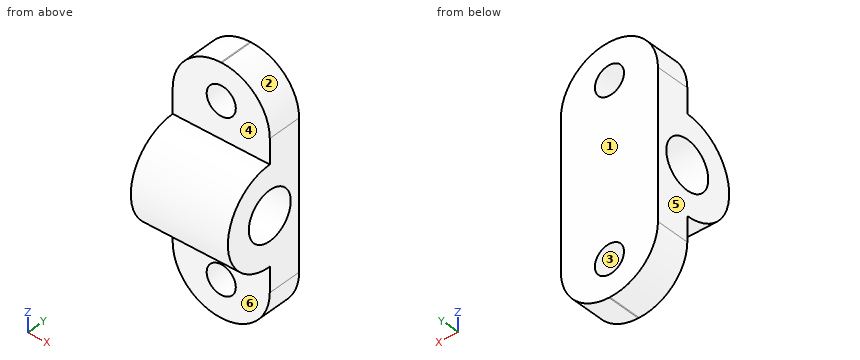
from build123d import *

# Parameters (mm, degrees)
PAD030_DEPTH             = 20
SKETCH021_R              = 5
POCKET001006_DEPTH       = 20.001
FILLET_R                 = 9.9
SKETCH024_R              = 3
POCKET002_DEPTH          = 7.001
CLONE076_ROLL_ANGLE      = 90
CLONE076_PLACEMENT_ANGLE = -90


with BuildPart() as part:
    # Sketch020 → Pad030 (new body)
    with BuildSketch(Plane.XY):
        with BuildLine():
            Line((18, 0), (25, 0))
            Line((25, 0), (25, 15))
            ThreePointArc((25, 15), (35, 25), (25, 35))
            Line((25, 35), (25, 50))
            Line((25, 50), (18, 50))
            Line((18, 50), (18, 0))
        make_face()
    extrude(amount=PAD030_DEPTH)

    # Sketch021 → Pocket001006 (cut, through all)
    with BuildSketch(Plane(origin=(0, 0, 0), x_dir=(1, 0, 0), z_dir=(0, 0, -1))):
        with Locations((25, -25)):
            Circle(SKETCH021_R)
    extrude(amount=-POCKET001006_DEPTH, mode=Mode.SUBTRACT)

    # Fillet
    fillet_edges = [part.edges().sort_by_distance(p)[0] for p in [
        (21.5, 0, 0),
        (21.5, 50, 0),
        (21.5, 50, 20),
        (21.5, 0, 20),
    ]]
    fillet(fillet_edges, radius=FILLET_R)

    # Sketch024 → Pocket002 (cut, through all)
    with BuildSketch(Plane.YZ.offset(25)):
        with Locations((7.5, 10)):
            Circle(SKETCH024_R)
        with Locations((42.5, 10)):
            Circle(SKETCH024_R)
    extrude(amount=-POCKET002_DEPTH, mode=Mode.SUBTRACT)


with BuildPart() as part_1:
    # Clone076 roll: moved
    add(part.part.rotate(Axis((0, 0, 0), (1, 0, 0)), CLONE076_ROLL_ANGLE))


with BuildPart() as part_2:
    # Clone076 placement: moved
    add(part_1.part.moved(Location((120.75, 1500, 0))).rotate(Axis((120.75, 1500, 0), (0, 0, 1)), CLONE076_PLACEMENT_ANGLE))


with BuildPart() as part_3:
    # Clone078 placement: moved
    add(part_2.part.moved(Location((347.25, 0, 0))))


solid = part_3.part
Can you work these out from the model? Positions are in its coordinate system, mm. Face numbers are marked on the shaded views. A direction names the side the tool comes from. Give positions to 0.01 mm unless a question says otherwise; leave off trailing zeros. Order: outer loops, then holes, each group sorted by start corner. A loop starts at its lowest first (then second) coordinate and runs counter-clockwise, first axis right, second up. Notation, with made-up numbers: M -19.5,34.5 L 22.5,34.5 A35 cw 22.5,69.5 Z; hole C 9.5,-37.5 d11. An arc over 180 degrees is marked long. Use a Markdown table: item, result. Add a question column.
Item 1: Will these pins go through, and if not, where does the flat tip stop? pin 1 (4.5 mm diameter, centred on x = 454.5, z = 39.5, fed in from -Y); pin 2 (3.5 mm diameter, centred on x = 458, z = 42.5, fed in from -Y); pin 3 (3 mm diameter, centred on x = 455, y = 1468.5, fed in from +Z); pin 4 (6 mm diameter, centred on x = 452.5, y = 1478, fed in from +Z).
Item 2: Suppose I cut it at D-D (y = 1480.75). List the corners of the cut face in (x, z) for me, then the cut area to 3 significant figures.
Item 3: Suppose I cut it at C-C (x = 462.25). List the corners of the cut face in (y, z) for me.
Item 4: If I drill on L1, parallel to Z at x = 458, y = 1477.5; L2, parallel to Z at x = 458, y = 1479.25; L3, parallel to Y at x = 456.75, z = 25, over which ranges is the centre line in solid material (lowest first)? Write a range as [from, to].
Item 5: For the marked faces 4, 5 and 6, which set-ups out of +Z, -Z, +X, -X, +Y, -Y let a thin tool reach every point of the face, with its end or its side?
Item 6: We'd pull the mould along Z, two halves only. Please class the marked faces 1, 2 and 3: +Z half, -Z half, draft (parallel to the pull), parting line (faces both ways), or undercut.
Item 7: Suppose I cut it at A-A (y = 1476). List the corners of the cut face in (x, z) for me.
Item 8: Suppose I cut it at B-B (z = 25). List the corners of the cut face in (x, y) for me, then the cut area to 3 significant figures.
Answer sheet:
| question | item | result |
|---|---|---|
| 1 | pin 1 | stops at y = 1475 |
| 1 | pin 2 | passes through |
| 1 | pin 3 | stops at z = 33.66 |
| 1 | pin 4 | stops at z = 49.7 |
| 2 | outline | M 448,9.9 A9.9 ccw 457.9,0 L 458.1,0 A9.9 ccw 468,9.9 L 468,40.1 A9.9 ccw 458.1,50 L 457.9,50 A9.9 ccw 448,40.1 Z; hole C 458,7.5 d6; hole C 458,42.5 d6 |
| 2 | area | 859 mm² |
| 3 | outline | M 1475,0.91 L 1482,0.91 L 1482,49.09 L 1475,49.09 L 1475,35 A10 ccw 1475,15 Z; hole C 1475,25 d10 |
| 4 | L1 | z = [0, 4.5], [10.5, 20.67], [29.33, 39.5], [45.5, 50] |
| 4 | L2 | z = [0, 4.5], [10.5, 22.37], [27.63, 39.5], [45.5, 50] |
| 4 | L3 | y = [1465, 1470], [1480, 1482] |
| 5 | face 4 | +Z, +X, -X, -Y |
| 5 | face 5 | +Z, -Z, -X, +Y, -Y |
| 5 | face 6 | -Z, +X, -X, -Y |
| 6 | face 1 | draft |
| 6 | face 2 | +Z half |
| 6 | face 3 | undercut |
| 7 | outline | M 448,9.9 A9.9 ccw 457.9,0 L 458.1,0 A9.9 ccw 468,9.9 L 468,20.1 L 448,20.1 Z; M 448,29.9 L 468,29.9 L 468,40.1 A9.9 ccw 458.1,50 L 457.9,50 A9.9 ccw 448,40.1 Z; hole C 458,7.5 d6; hole C 458,42.5 d6 |
| 8 | outline | M 448,1465 L 468,1465 L 468,1470 L 448,1470 Z; M 448,1480 L 468,1480 L 468,1482 L 448,1482 Z |
| 8 | area | 140 mm² |
